Design review of the part built by this model. Coordinates are the model's own, in mm. A direction names the side the tool comes from. Give positions to 0.01 mm unless a question says otherwise; leave off trailing zeros. Write each loop counter-clockwise with the first axis right and the second up, starting at its lowest first coordinate (ties: lowest second). Pieces come first, ordered by that corner, then holes.
```python
from build123d import *

# Parameters (mm, degrees)
SKETCH1_W                       = 15
SKETCH1_H                       = 15
BOSS_EXTRUDE1_DEPTH             = 93
SKETCH2_R                       = 3
BOSS_EXTRUDE2_DEPTH             = 7
FILLET1_R                       = 2
BOSS_EXTRUDE3_DEPTH             = 1
BOSS_EXTRUDE3_DEPTH_BACK        = 4
SKETCH5_W                       = 1.2
SKETCH5_H                       = 17
SKETCH6_W                       = 4.3
SKETCH6_H                       = 20
BOSS_EXTRUDE4_DEPTH             = 1.2
BOSS_EXTRUDE5_REACH             = 106.522
SKETCH9_W                       = 1.9
SKETCH9_H                       = 20
CUT_EXTRUDE2_DEPTH              = 17
SKETCH10_R                      = 1.75
CUT_EXTRUDE3_DEPTH              = 10
SKETCH11_W                      = 1
SKETCH11_H                      = 3
BOSS_EXTRUDE6_DEPTH             = 15
BOSS_EXTRUDE7_REACH             = 79.176
SKETCH12_W                      = 15
SKETCH12_H                      = 1
BOSS_EXTRUDE7_DIRECTION_2_REACH = 79.176
SKETCH3_W                       = 3.2
SKETCH3_H                       = 2.1
CUT_EXTRUDE1_DEPTH              = 105.263560269
BOSS_EXTRUDE8_DEPTH             = 5


with BuildPart() as part:
    # Sketch1 → Boss-Extrude1 (new body)
    with BuildSketch(Plane(origin=(0, 0, 0), x_dir=(1, 0, 0), z_dir=(0, 1, 0))):
        Rectangle(SKETCH1_W, SKETCH1_H)
    extrude(amount=BOSS_EXTRUDE1_DEPTH)

    # Sketch2 → Boss-Extrude2 (add)
    with BuildSketch(Plane(origin=(0, 93, 0), x_dir=(1, 0, 0), z_dir=(0, 1, 0))):
        with Locations(Location((1.5, -2.5, 0), (0, 0, 90))):
            Circle(SKETCH2_R)
    extrude(amount=BOSS_EXTRUDE2_DEPTH)

    # Fillet1
    fillet1_edges = [part.edges().sort_by_distance(p)[0] for p in [
        (7.5, 46.5, 7.5),
    ]]
    fillet(fillet1_edges, radius=FILLET1_R)

    # Sketch5 → Boss-Extrude3 (add, two sides: drawn at the far end of the back side and taken through both)
    with BuildSketch(Plane(origin=(0, 0, -7.5), x_dir=(-1, 0, 0), z_dir=(0, 0, -1)).offset(-BOSS_EXTRUDE3_DEPTH_BACK)):
        Polygon((-21.7, 24), (-7.5, 24), (-7.5, 27), (-17.4, 27), (-18.6, 27), (-20.5, 27), (-20.5, 44), (-21.7, 44), align=None)
        with Locations((-18, 35.5)):
            Rectangle(SKETCH5_W, SKETCH5_H)
    extrude(amount=BOSS_EXTRUDE3_DEPTH + BOSS_EXTRUDE3_DEPTH_BACK)

    # Sketch6 → Boss-Extrude4 (add)
    with BuildSketch(Plane.XY.offset(-3.5)):
        with Locations((19.55, 34)):
            Rectangle(SKETCH6_W, SKETCH6_H)
    extrude(amount=-BOSS_EXTRUDE4_DEPTH)

    # Boss-Extrude5: up to this face of the body (flat: up to its plane)
    boss_extrude5_end = Plane(part.part.faces().sort_by_distance((17.4, 35.5, -6))[0])
    # Sketch7 → Boss-Extrude5 (add, up to the picked face)
    with BuildSketch(Plane(origin=(21.7, 0, 0), x_dir=(0, 0, -1), z_dir=(1, 0, 0)), mode=Mode.PRIVATE) as boss_extrude5_sk1:
        Polygon((5.5, 34.5), (5.5, 44), (8.5, 44), (8.5, 37.74), (12.5, 37.74), (12.5, 31.5), (8.5, 31.5), align=None)
    boss_extrude5_tool1 = split(extrude(boss_extrude5_sk1.sketch, amount=-BOSS_EXTRUDE5_REACH, mode=Mode.PRIVATE), bisect_by=boss_extrude5_end, keep=Keep.BOTH, mode=Mode.PRIVATE)
    add(boss_extrude5_tool1.solids().sort_by(Axis((21.7, 36.8097, -8.546066), (-1, 0, 0)))[0])

    # Sketch9 → Cut-Extrude2 (cut)
    with BuildSketch(Plane(origin=(0, 44, 0), x_dir=(1, 0, 0), z_dir=(0, 1, 0))):
        with Locations((19.55, 14.7)):
            Rectangle(SKETCH9_W, SKETCH9_H)
    extrude(amount=-CUT_EXTRUDE2_DEPTH, mode=Mode.SUBTRACT)

    # Sketch10 → Cut-Extrude3 (cut)
    with BuildSketch(Plane(origin=(21.7, 0, 0), x_dir=(0, 0, -1), z_dir=(1, 0, 0))):
        with Locations(Location((8.46, 34.62, 0), (0, 0, 90))):
            Circle(SKETCH10_R)
    extrude(amount=-CUT_EXTRUDE3_DEPTH, mode=Mode.SUBTRACT)

    # Sketch11 → Boss-Extrude6 (add)
    with BuildSketch(Plane.ZY.offset(-7.5)):
        with Locations((-8, 25.5)):
            Rectangle(SKETCH11_W, SKETCH11_H)
    extrude(amount=BOSS_EXTRUDE6_DEPTH)

    # Boss-Extrude7: up to this face of the body (flat: up to its plane)
    boss_extrude7_end = Plane(part.part.faces().sort_by_distance((-0.247443472, 93, -0.391798042))[0])
    # Sketch12 → Boss-Extrude7 (add, up to the picked face)
    with BuildSketch(Plane(origin=(0, 27, 0), x_dir=(1, 0, 0), z_dir=(0, 1, 0)), mode=Mode.PRIVATE) as boss_extrude7_sk1:
        with Locations((0, 8)):
            Rectangle(SKETCH12_W, SKETCH12_H)
    boss_extrude7_tool1 = split(extrude(boss_extrude7_sk1.sketch, amount=BOSS_EXTRUDE7_REACH, mode=Mode.PRIVATE), bisect_by=boss_extrude7_end, keep=Keep.BOTH, mode=Mode.PRIVATE)
    add(boss_extrude7_tool1.solids().sort_by(Axis((0, 27, -8), (0, 1, 0)))[0])

    # Boss-Extrude7 direction 2: up to this face of the body (flat: up to its plane)
    boss_extrude7_direction_2_end = Plane(part.part.faces().sort_by_distance((-0.027012272, 0, -0.027012272))[0])
    # Sketch12 → Boss-Extrude7 direction 2 (add, up to the picked face)
    with BuildSketch(Plane(origin=(0, 27, 0), x_dir=(1, 0, 0), z_dir=(0, 1, 0)), mode=Mode.PRIVATE) as boss_extrude7_direction_2_sk1:
        with Locations((0, 8)):
            Rectangle(SKETCH12_W, SKETCH12_H)
    boss_extrude7_direction_2_tool1 = split(extrude(boss_extrude7_direction_2_sk1.sketch, amount=-BOSS_EXTRUDE7_DIRECTION_2_REACH, mode=Mode.PRIVATE), bisect_by=boss_extrude7_direction_2_end, keep=Keep.BOTH, mode=Mode.PRIVATE)
    add(boss_extrude7_direction_2_tool1.solids().sort_by(Axis((0, 27, -8), (0, -1, 0)))[0])

    # Sketch3 → Cut-Extrude1 (cut, through all)
    with BuildSketch(Plane.XY.offset(7.5)):
        with Locations((-5.9, 11.05)):
            Rectangle(SKETCH3_W, SKETCH3_H)
    extrude(amount=-CUT_EXTRUDE1_DEPTH, mode=Mode.SUBTRACT)

    # Sketch13 → Boss-Extrude8 (add)
    with BuildSketch(Plane.XY.offset(-3.5)):
        Polygon((21.7, 24), (7.5, 24), (7.5, 9.8), align=None)
    extrude(amount=-BOSS_EXTRUDE8_DEPTH)


solid = part.part
```
(1) To check wall thickness, follow L1, parallel to Z at x = 18.1, y = 34.62; L2, parallel to Z at x = -6, y = 30; L3, parallel to X at y = 22, z = -2. State the ranges of each line that lie inside material, in increasing order.
Resolved:
L1: z = -12.5 to -10.21, -6.71 to -3.5
L2: z = -8.5 to 7.5
L3: x = -7.5 to 7.5
(2) Consider section A-A, the plane y = 34.62. Give the boundary of the cut face in (x, z), then the cut area to 3 significant figures.
Resolved:
outline: (-7.5, -8.5) - (7.5, -8.5) - (7.5, 5.5) arc R2 ccw to (5.5, 7.5) - (-7.5, 7.5) - close; (17.4, -12.5) - (18.6, -12.5) - (18.6, -10.21) - (17.4, -10.21) - close; (17.4, -6.71) - (18.6, -6.71) - (18.6, -4.7) - (20.5, -4.7) - (20.5, -6.71) - (21.7, -6.71) - (21.7, -3.5) - (17.4, -3.5) - close; (20.5, -12.5) - (21.7, -12.5) - (21.7, -10.21) - (20.5, -10.21) - close
area: 255 mm2
(3) Consider section C-C, the plane y = 68. Give the boundary of the cut face in (x, z).
Resolved:
outline: (-7.5, -8.5) - (7.5, -8.5) - (7.5, 5.5) arc R2 ccw to (5.5, 7.5) - (-7.5, 7.5) - close
(4) Consider section B-B, the plane z = 2.5. Give the boundary of the cut face in (x, y).
Resolved:
outline: (-7.5, 0) - (7.5, 0) - (7.5, 93) - (4.5, 93) - (4.5, 100) - (-1.5, 100) - (-1.5, 93) - (-7.5, 93) - (-7.5, 12.1) - (-4.3, 12.1) - (-4.3, 10) - (-7.5, 10) - close
(5) Mouldability with a two-part tool opening along X and no side actions: class faces 6 (the face through (20, 27, -7)), 7 (the face through (-4.3, 11, 0)), 8 (the face through (-1, 46, 7.5)), 9 (the face through (18.6, 35, -6)) as pulls with the +X half, pulls with the -X half, needs draft (parallel to the pull), parting line crosses it, or undercut.
Resolved:
face 6: undercut
face 7: pulls with the -X half
face 8: needs draft
face 9: undercut
(6) Consider section D-D, the plane x = 1.5. Give the boundary of the cut face in (y, z), then the cut area to 3 significant figures.
Resolved:
outline: (0, -8.5) - (93, -8.5) - (93, -0.5) - (100, -0.5) - (100, 5.5) - (93, 5.5) - (93, 7.5) - (0, 7.5) - close
area: 1,530 mm2
(7) Clearance check with flat-ended pins moving along their axes: P1, Ø1.1, axis at y = 11, z = -0.5, coming from the -X side; P2, Ø2, axis at x = 20, z = -6.5, coming from the +Y side; P3, Ø0.9, axis at x = 19.5, y = 36, coming from the -Z side; P4, Ø1, axis at x = 8.5, y = 84, coming from the +Z side. State where each tip first meets the part, or that it passes through.
Resolved:
P1: stops at x = -4.3
P2: stops at y = 44
P3: stops at z = -4.7
P4: passes through
(8) Tool access review of faces 1 (the face through (18, 44, -5)), 2 (the face through (-6, 12.1, 0)), 3 (the face through (13, 27, -6)), 4 (the face through (20, 36, -4.7)), 5 (the face through (18, 27, -3.5)): name each direction out of +Z, -Z, +X, -X, +Y, -Y from which nothing blocks a thin tool from reaching the whole face with its end or side.
Resolved:
face 1: +Z, -Z, +X, +Y
face 2: +Z, -Z, -X
face 3: +Z, -Z, +Y
face 4: -Z, +Y
face 5: +Z, +X, +Y, -Y
